Model file for the job. Use its own axes, mm. A direction names the side the tool comes from. Round coordinates to 2 decimals unless told otherwise and drop trailing zeros. Order: outer loops, then holes, each group sorted by start corner. A loop starts at its lowest first (then second) coordinate and runs counter-clockwise, first axis right, second up. Notation, with made-up numbers: (-1.5, -34.75) -> (23.5, -34.75) arc R17 ccw to (23.5, -21.75) -> close; hole circle Ø4 at (-20.5, -20.5). An arc over 180 degrees is marked (long way). Put each result on its own line as item: value. Start each with the question number.
Q1. Cut at B-B, the plane x = -8.5. List the corners of the cut face in (y, z), and give its area (3 significant figures).
Q2. Probe L1, parallel to Z at x = -85.5, y = 33.5; L2, parallel to X at y = 40, z = -3; L3, parallel to Z at x = -86, y = 8.5. List the from-to ranges inside material, lowest first.
Q3. 3-axis set-ups, long thin cutter, end or side, ignore diameter. For faces 1 (the face through (49.886, 20.706, 38.267)), 2 (the face through (43, 27, -19)), 3 (the face through (43, 13, -16.452)): which of +Z, -Z, +X, -X, +Y, -Y reach the whole face in a straight line?
Q4. Cut at A-A, the plane z = -15. List the corners of the cut face in (x, y).
Q5. Flat gauge pins, fed straight in: P1, Ø4.5, axis at x = -89.71, z = 31.55, coming from the -Y side; P2, Ø3, axis at x = -89.71, z = -21.45, coming from the +Y side; P3, Ø3, axis at x = 41, z = 29.5, coming from the +Y side. Where does each tip first touch, or does it go through?
Q6. Cut at C-C, the plane y = 19.5. List the corners of the cut face in (x, z).
Q7. Pull direction Z, two halves, no side cores. Call faces 4 (the face through (-24, 42, -27)), 5 (the face through (-96.303, 20.706, -28.171)), 6 (the face through (45.2, 13.31, -22.05)): released by +Z, released by -Z, zero draft, split by the parting line, or undercut.
from build123d import *

# Parameters (mm, degrees)
SKETCH1_W             = 10
SKETCH1_H             = 10
SKETCH1_R             = 2
BOSS_EXTRUDE5_DEPTH   = 27
BOSS_EXTRUDE5_2_DEPTH = 27
BOSS_EXTRUDE5_3_DEPTH = 27
BOSS_EXTRUDE5_4_DEPTH = 27
SKETCH1_7_W           = 143
SKETCH1_7_H           = 63
BOSS_EXTRUDE6_DEPTH   = 42


with BuildPart() as part:
    # Sketch1 → Boss-Extrude5 (new body)
    with BuildSketch(Plane(origin=(0, 0, 0), x_dir=(1, 0, 0), z_dir=(0, 1, 0))):
        with Locations((-89.708361573, 21.452000773)):
            Rectangle(SKETCH1_W, SKETCH1_H)
        with Locations((-89.708361573, 21.452000773)):
            Circle(SKETCH1_R, mode=Mode.SUBTRACT)
    extrude(amount=BOSS_EXTRUDE5_DEPTH)



with BuildPart() as body_2:
    # Sketch1 → Boss-Extrude5 2 (new body)
    with BuildSketch(Plane(origin=(0, 0, 0), x_dir=(1, 0, 0), z_dir=(0, 1, 0))):
        with Locations((-89.708361573, -31.547999227)):
            Rectangle(SKETCH1_W, SKETCH1_H)
        with Locations((-89.708361573, -31.547999227)):
            Circle(SKETCH1_R, mode=Mode.SUBTRACT)
    extrude(amount=BOSS_EXTRUDE5_2_DEPTH)


with BuildPart() as body_3:
    # Sketch1 → Boss-Extrude5 3 (new body)
    with BuildSketch(Plane(origin=(0, 0, 0), x_dir=(1, 0, 0), z_dir=(0, 1, 0))):
        with Locations((43.291638427, -31.547999227)):
            Rectangle(SKETCH1_W, SKETCH1_H)
        with Locations((43.291638427, -31.547999227)):
            Circle(SKETCH1_R, mode=Mode.SUBTRACT)
    extrude(amount=BOSS_EXTRUDE5_3_DEPTH)


with BuildPart() as body_4:
    # Sketch1 → Boss-Extrude5 4 (new body)
    with BuildSketch(Plane(origin=(0, 0, 0), x_dir=(1, 0, 0), z_dir=(0, 1, 0))):
        with Locations((43.291638427, 21.452000773)):
            Rectangle(SKETCH1_W, SKETCH1_H)
        with Locations((43.291638427, 21.452000773)):
            Circle(SKETCH1_R, mode=Mode.SUBTRACT)
    extrude(amount=BOSS_EXTRUDE5_4_DEPTH)


with BuildPart() as part_1:
    add(part.part)

    add(body_2.part)  # Boss-Extrude6 merges body 2

    add(body_3.part)  # Boss-Extrude6 merges body 3

    add(body_4.part)  # Boss-Extrude6 merges body 4
    # Sketch1_7 → Boss-Extrude6 (add)
    with BuildSketch(Plane(origin=(0, 0, 0), x_dir=(1, 0, 0), z_dir=(0, 1, 0))):
        with BuildLine():
            Line((-98.708361573, 22.452000773), (-98.708361573, -32.547999227))
            ThreePointArc((-98.708361573, -32.547999227), (-96.365215823, -38.204853476), (-90.708361573, -40.547999227))
            Line((-90.708361573, -40.547999227), (44.291638427, -40.547999227))
            ThreePointArc((44.291638427, -40.547999227), (49.948492676, -38.204853476), (52.291638427, -32.547999227))
            Line((52.291638427, -32.547999227), (52.291638427, 22.452000773))
            ThreePointArc((52.291638427, 22.452000773), (49.948492676, 28.108855023), (44.291638427, 30.452000773))
            Line((44.291638427, 30.452000773), (-90.708361573, 30.452000773))
            ThreePointArc((-90.708361573, 30.452000773), (-96.365215823, 28.108855023), (-98.708361573, 22.452000773))
        make_face()
        with Locations((-23.208361573, -5.047999227)):
            Rectangle(SKETCH1_7_W, SKETCH1_7_H, mode=Mode.SUBTRACT)
    extrude(amount=BOSS_EXTRUDE6_DEPTH)


solid = part_1.part
Ans:
1. outline: (0, -30.45) -> (42, -30.45) -> (42, -26.45) -> (0, -26.45) -> close; (0, 36.55) -> (42, 36.55) -> (42, 40.55) -> (0, 40.55) -> close
1. area: 336 mm^2
2. L1: z = -30.45 to -26.45, 36.55 to 40.55
2. L2: x = -98.71 to -94.71, 48.29 to 52.29
2. L3: z = -30.45 to -16.45, 26.55 to 40.55
3. face 1: +Z, +X, +Y, -Y
3. face 2: +Y
3. face 3: +Y, -Y
4. outline: (-98.71, 0) -> (-94.71, 0) -> (-94.71, 42) -> (-98.71, 42) -> close; (48.29, 0) -> (52.29, 0) -> (52.29, 42) -> (48.29, 42) -> close
5. P1: stops at y = 0
5. P2: passes through
5. P3: stops at y = 27
6. outline: (-98.71, -22.45) arc R8 ccw to (-90.71, -30.45) -> (44.29, -30.45) arc R8 ccw to (52.29, -22.45) -> (52.29, 32.55) arc R8 ccw to (44.29, 40.55) -> (-90.71, 40.55) arc R8 ccw to (-98.71, 32.55) -> close; hole (-94.71, -16.45) -> (-84.71, -16.45) -> (-84.71, -26.45) -> (38.29, -26.45) -> (38.29, -16.45) -> (48.29, -16.45) -> (48.29, 26.55) -> (38.29, 26.55) -> (38.29, 36.55) -> (-84.71, 36.55) -> (-84.71, 26.55) -> (-94.71, 26.55) -> close; hole circle Ø4 at (-89.71, -21.45); hole circle Ø4 at (-89.71, 31.55); hole circle Ø4 at (43.29, -21.45); hole circle Ø4 at (43.29, 31.55)
7. face 4: zero draft
7. face 5: released by -Z
7. face 6: undercut
